Input: part model. Units: mm. Frame: model coordinates. Face numbers are marked on the shaded views. A direction names the side the tool comes from. Round coordinates to 2 decimals unless told otherwise and drop trailing zeros. Loops run counter-clockwise (first coordinate to the right, second up) from the corner with the lowest first, then second, coordinate; pieces in that order, holes last.
(1) Access query for the marked faces 4 and 5. Directions: +Z, -Z, +X, -X, +Y, -Y. A direction counts if a zero-diameter tool reaches every point of the face in a straight line with its end or side. Return the directions, or none.
(2) Line query: line 1 (Y direction, x = 2, z = 21); line 2 (Z direction, x = 4, y = 18.45); line 3 (Z direction, x = 4, y = 19.45). Output: solid intervals per line, ascending.
(3) Cut plane C-C, the plane z = 11.75. Output: boundary loops of the cut face in (x, y).
(4) Cut plane A-A, the plane x = 4. Output: boundary loops of the cut face in (y, z).
(5) First-contact query: pin 1 Ø1 at (y, z) = (16.5, 25) entering from -X; pin 2 Ø12 at (x, y) = (16.5, 10.5) entering from +Z. Flat tips, straight axial feed; report the tip coordinate or a pass-through.
(6) Draft query along Y for the marked faces 1, 2 and 3. Return one class per face: released by +Y, released by -Y, zero draft, split by the parting line, or undercut.
(7) Cut plane D-D, the plane x = 1.5. Output: boundary loops of the cut face in (y, z), and give its area (3 significant figures).
(8) Cut plane B-B, the plane z = 8.75. Output: boundary loops of the cut face in (x, y).
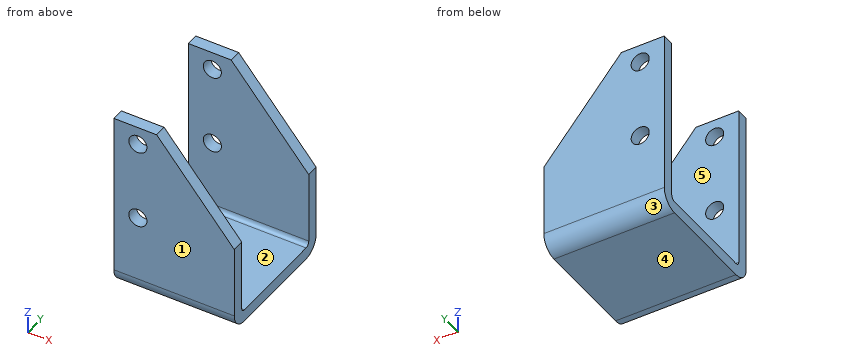
from build123d import *

# Parameters (mm, degrees)
SCHIZZO1_W                       = 20
SCHIZZO1_H                       = 18
BASE_FLANGIA1_DEPTH              = 2
BORDO_FLANGIA3_STRIP_W           = 9.4732
BORDO_FLANGIA3_STRIP_H           = 2
BORDO_FLANGIA3_STRIP_CUT_DEPTH   = 20
BORDO_FLANGIA3_STRIP_2_W         = 9.4732
BORDO_FLANGIA3_STRIP_2_H         = 2
BORDO_FLANGIA3_STRIP_CUT_2_DEPTH = 20
BORDO_FLANGIA3_DEPTH             = 20
BORDO_FLANGIA3_BEND_DEPTH        = 20
TAGLIO_ESTRUSIONE1_DEPTH         = 41.841155713
TAGLIO_ESTRUSIONE1_DEPTH_BACK    = 41.841155713
TAGLIO_ESTRUSIONE2_DEPTH         = 41.841155713
TAGLIO_ESTRUSIONE2_DEPTH_BACK    = 41.841155713
SCHIZZO20_R                      = 1.5


# Sheet-metal steps are written as plain solids
with BuildPart() as part:
    # Schizzo1 → Base-Flangia1 (new body)
    with BuildSketch(Plane.XY):
        with Locations((10, 9)):
            Rectangle(SCHIZZO1_W, SCHIZZO1_H)
    extrude(amount=-BASE_FLANGIA1_DEPTH)

    # Bordo-Flangia3 strip (across the edge) → Bordo-Flangia3 strip cut (cut)
    with BuildSketch(Plane(origin=(20, 18, 0), x_dir=(0, -1, 0), z_dir=(-1, 0, 0))):
        with Locations((-4, -1)):
            Rectangle(BORDO_FLANGIA3_STRIP_W, BORDO_FLANGIA3_STRIP_H)
    extrude(amount=BORDO_FLANGIA3_STRIP_CUT_DEPTH, mode=Mode.SUBTRACT)

    # Bordo-Flangia3 strip 2 (across the edge) → Bordo-Flangia3 strip cut 2 (cut)
    with BuildSketch(Plane.YZ):
        with Locations((-4, -1)):
            Rectangle(BORDO_FLANGIA3_STRIP_2_W, BORDO_FLANGIA3_STRIP_2_H)
    extrude(amount=BORDO_FLANGIA3_STRIP_CUT_2_DEPTH, mode=Mode.SUBTRACT)

    # Bordo-Flangia3 section (across the edge) → Bordo-Flangia3 (add)
    with BuildSketch(Plane(origin=(20, 18, 0), x_dir=(0, -1, 0), z_dir=(-1, 0, 0))):
        with BuildLine():
            Line((-2, 0.7366), (-2, 28))
            Line((-2, 28), (0, 28))
            Line((0, 28), (0, 0.7366))
            ThreePointArc((0, 0.7366), (0.215745145, 0.215745145), (0.7366, 0))
            Line((0.7366, 0), (0.7366, -2))
            ThreePointArc((0.7366, -2), (-1.198468417, -1.198468417), (-2, 0.7366))
        make_face()
    extrude(amount=BORDO_FLANGIA3_DEPTH)

    # Bordo-Flangia3 section 2 (across the edge) → Bordo-Flangia3 bend (add)
    with BuildSketch(Plane.YZ):
        with BuildLine():
            Line((-2, 0.7366), (-2, 28))
            Line((-2, 28), (0, 28))
            Line((0, 28), (0, 0.7366))
            ThreePointArc((0, 0.7366), (0.215745145, 0.215745145), (0.7366, 0))
            Line((0.7366, 0), (0.7366, -2))
            ThreePointArc((0.7366, -2), (-1.198468417, -1.198468417), (-2, 0.7366))
        make_face()
    extrude(amount=BORDO_FLANGIA3_BEND_DEPTH)

    # Schizzo19 → Taglio-Estrusione1 (cut, two sides: drawn at the far end of the back side and taken through both)
    with BuildSketch(Plane.XZ.offset(2).offset(-TAGLIO_ESTRUSIONE1_DEPTH_BACK)):
        Polygon((7.119394424, 28), (20, 12.7), (20, 28), align=None)
    extrude(amount=TAGLIO_ESTRUSIONE1_DEPTH + TAGLIO_ESTRUSIONE1_DEPTH_BACK, mode=Mode.SUBTRACT)

    # Schizzo20 → Taglio-Estrusione2 (cut, two sides: drawn at the far end of the back side and taken through both)
    with BuildSketch(Plane(origin=(0, 20, 0), x_dir=(1, 0, 0), z_dir=(0, 1, 0)).offset(-TAGLIO_ESTRUSIONE2_DEPTH_BACK)):
        with Locations(Location((4, -11.7366, 0), (0, 0, 270))):
            Circle(SCHIZZO20_R)
        with Locations(Location((4, -25, 0), (0, 0, 270))):
            Circle(SCHIZZO20_R)
    extrude(amount=TAGLIO_ESTRUSIONE2_DEPTH + TAGLIO_ESTRUSIONE2_DEPTH_BACK, mode=Mode.SUBTRACT)


solid = part.part
Reported:
1. face 4: -Z, +X, -X, +Y, -Y
1. face 5: +Z, +X, -X
2. line 1: y = -2 to 0, 18 to 20
2. line 2: z = -1.73 to 10.24, 13.24 to 23.5, 26.5 to 28
2. line 3: z = -0.91 to 10.24, 13.24 to 23.5, 26.5 to 28
3. outline: (0, -2) - (2.5, -2) - (2.5, 0) - (0, 0) - close; (0, 18) - (2.5, 18) - (2.5, 20) - (0, 20) - close; (5.5, -2) - (20, -2) - (20, 0) - (5.5, 0) - close; (5.5, 18) - (20, 18) - (20, 20) - (5.5, 20) - close
4. outline: (-2, 0.74) arc R2.74 ccw to (0.74, -2) - (17.26, -2) arc R2.74 ccw to (20, 0.74) - (20, 10.24) - (18, 10.24) - (18, 0.74) arc R0.74 cw to (17.26, 0) - (0.74, 0) arc R0.74 cw to (0, 0.74) - (0, 10.24) - (-2, 10.24) - close; (-2, 13.24) - (0, 13.24) - (0, 23.5) - (-2, 23.5) - close; (-2, 26.5) - (0, 26.5) - (0, 28) - (-2, 28) - close; (18, 13.24) - (20, 13.24) - (20, 23.5) - (18, 23.5) - close; (18, 26.5) - (20, 26.5) - (20, 28) - (18, 28) - close
5. pin 1: passes through
5. pin 2: stops at z = 0
6. face 1: released by -Y
6. face 2: undercut
6. face 3: released by +Y
7. outline: (-2, 0.74) arc R2.74 ccw to (0.74, -2) - (17.26, -2) arc R2.74 ccw to (20, 0.74) - (20, 28) - (18, 28) - (18, 0.74) arc R0.74 cw to (17.26, 0) - (0.74, 0) arc R0.74 cw to (0, 0.74) - (0, 28) - (-2, 28) - close
7. area: 153 mm2
8. outline: (0, -2) - (20, -2) - (20, 0) - (0, 0) - close; (0, 18) - (20, 18) - (20, 20) - (0, 20) - close
